Autodesk Inventor part; units mm, degrees
ref_plane "YZ Plane" through (0, 0, 0) normal (1, 0, 0) x (0, 1, 0)
ref_plane "XZ Plane" through (0, 0, 0) normal (0, 1, 0) x (-1, 0, 0)
ref_plane "XY Plane" through (0, 0, 0) normal (0, 0, 1) x (1, 0, 0)
sketch "Sketch1" plane through (0, 0, 0) normal (0, 1, 0) x (-1, 0, 0)
  line L0 (0, 0) -> (-20, 0)
  line L1 (-20, 0) -> (-20, -100)
  line L2 (-20, -100) -> (0, -100)
  line L3 (0, -100) -> (0, 0)
  dimension "d0" = 20
  dimension "d1" = 100
extrude "Extrusion1" add sketch "Sketch1" along normal blind 15
sketch "Sketch2" plane through (0, 15, 0) normal (0, 1, 0) x (1, 0, 0)
  line L0 (20, 0) -> (20, 100)
  line L1 (0, 100) -> (0, 0)
  line L2 (20, 0) -> (0, 0)
  line L3 (0, 0) -> (0, 19.5)
  line L4 (0, 19.5) -> (20, 19.5)
  line L5 (20, 19.5) -> (20, 0)
  dimension "d4" = 19.5
extrude "Extrusion2" add sketch "Sketch2" along normal blind 15
sketch "Sketch3" plane through (0, 15, 0) normal (0, 1, 0) x (1, 0, 0)
  line L0 (20, 19.5) -> (0, 19.5)
  line L1 (0, 19.5) -> (0, 22.5)
  line L2 (0, 100) -> (0, 0)
  line L3 (0, 22.5) -> (3.0005, 19.5)
  line L4 (3.0005, 19.5) -> (0, 19.5)
  line L5 (20, 19.5) -> (20, 22.5)
  line L6 (20, 0) -> (20, 100)
  line L7 (20, 22.5) -> (16.9995, 19.5)
  line L8 (16.9995, 19.5) -> (20, 19.5)
  dimension "d7" = 3
  dimension "d8" = 4.243
  dimension "d9" = 3
  dimension "d10" = 4.243
extrude "Extrusion3" add sketch "Sketch3" along normal blind 15
sketch "Sketch4" plane through (0, 0, 0) normal (0, 0, 1) x (1, 0, 0)
  point P0 (0, 0)
sketch "Sketch5" plane through (0, 0, 0) normal (0, 0, 1) x (1, 0, 0)
  line L0 (0, 0) -> (20, 0)
  line L1 (20, 30) -> (16.9995, 30)
  line L2 (0, 0) -> (20, 0)
  line L3 (20, 0) -> (20, 30)
  line L4 (20, 30) -> (0, 30)
  line L5 (0, 30) -> (0, 0)
extrude "Extrusion4" add sketch "Sketch5" along normal blind 80
sketch "Sketch6" plane through (0, 0, 80) normal (0, 0, 1) x (1, 0, 0)
  line L0 (19, 3) -> (1, 3)
  line L1 (1, 3) -> (1, 12)
  line L2 (1, 12) -> (19, 12)
  line L3 (19, 12) -> (19, 3)
  line L4 (0, 30) -> (0, 0)
  line L5 (0, 0) -> (20, 0)
  dimension "d15" = 18
  dimension "d16" = 9
  dimension "d17" = 1
  dimension "d18" = 3
extrude "Extrusion5" cut sketch "Sketch6" against normal blind 160
sketch "Sketch7" plane through (0, 0, 0) normal (0, -1, 0) x (1, 0, 0)
  circle A0 centre (10, -89.5) radius 2.25
  circle A1 centre (10, -74.5) radius 2.25
  line L0 (20, -100) -> (0, -100)
  line L1 (0, -100) -> (0, 80)
  point P0 (0, 0)
  point P1 (10, -100)
  dimension "d21" = 4.5
  dimension "d22" = 4.5
  dimension "d23" = 10.5
  dimension "d24" = 10.5
  dimension "d25" = 10
  dimension "d26" = 10
extrude "Extrusion6" cut sketch "Sketch7" against normal blind 160
sketch "Sketch8" plane through (0, 0, -80) normal (0, 0, 1) x (1, 0, 0)
  line L0 (19, 3) -> (1, 3)
  line L1 (1, 12) -> (19, 12)
  line L2 (19, 3) -> (1, 3)
  line L3 (1, 3) -> (1, 12)
  line L4 (1, 12) -> (19, 12)
  line L5 (19, 12) -> (19, 3)
  point P0 (0, 0)
extrude "Extrusion7" add sketch "Sketch8" along normal blind 170
sketch "Sketch9" plane through (0, 30, 0) normal (0, 1, 0) x (1, 0, 0)
  point P0 (0, 0)
sketch "Sketch10" plane through (0, 0, 90) normal (0, 0, 1) x (1, 0, 0)
  line L0 (19, 3) -> (1, 3)
  line L1 (1, 12) -> (19, 12)
  line L2 (1, 3) -> (19, 3)
  line L3 (19, 3) -> (19, 12)
  line L4 (19, 12) -> (1, 12)
  line L5 (1, 12) -> (1, 3)
  point P0 (0, 0)
extrude "Extrusion8" cut sketch "Sketch10" against normal blind 185
sketch "Sketch11" plane through (0, 15, 0) normal (0, 1, 0) x (1, 0, 0)
  line L0 (0, 100) -> (0, -80)
  line L1 (20, -80) -> (20, 100)
  line L2 (0, 100) -> (20, 100)
  line L3 (20, 100) -> (20, 97.7472)
  line L4 (20, 97.7472) -> (0, 97.7472)
  line L5 (0, 97.7472) -> (0, 100)
  point P0 (0, 0)
  point P1 (0, 97.7472)
extrude "Extrusion9" cut sketch "Sketch11" against normal blind 185
sketch "Sketch12" plane through (0, 30, 0) normal (0, 1, 0) x (1, 0, 0)
  circle A0 centre (10, -70.4515) radius 30
  point P0 (0, 0)
  dimension "d35" = 60
extrude "Extrusion10" add sketch "Sketch12" along normal mid plane 60
sketch "Sketch13" plane through (10, 60, 70.4515) normal (0, 1, 0) x (1, 0, 0)
  circle A0 centre (0, 0) radius 30
  point P0 (-10, 70.4515)
extrude "Extrusion11" cut sketch "Sketch13" against normal blind 30
sketch "Sketch14" plane through (0, 30, 0) normal (0, 1, 0) x (1, 0, 0)
  point P0 (0, 0)
sketch "Sketch15" plane through (0, 0, 0) normal (0, -1, 0) x (1, 0, 0)
  arc A0 (1, 41.8333) -> (19, 41.8333) centre (10, 70.4515) ccw
  circle A1 centre (4.9424, 40.8809) radius 2.5
  circle A2 centre (15.0576, 40.8809) radius 2.5
  point P0 (0, 0)
  dimension "d40" = 5
  dimension "d41" = 5
extrude "Extrusion12" cut sketch "Sketch15" against normal blind 13
sketch "Sketch16" plane through (0, 0, 0) normal (0, -1, 0) x (1, 0, 0)
  circle A0 centre (10, -89.5) radius 2.25
  circle A1 centre (10, -89.5) radius 3.5
  circle A2 centre (10, -74.5) radius 2.25
  circle A3 centre (10, -74.5) radius 3.5
  point P0 (0, 0)
  dimension "d44" = 7
  dimension "d45" = 7
extrude "Extrusion13" cut sketch "Sketch16" against normal blind 6
fillet "Fillet1" radius 2 8 edges at (20, 30, 9.8336) (20, 15, -60.1236) (0, 15, -60.1236) (0, 30, 9.8336) (0, 0, -27.79) (20, 0, -27.79) (10, 30, 100.4515) (10, 0, 100.4515)
sketch "Sketch17" plane through (0, 0, 0) normal (0, -1, 0) x (1, 0, 0)
  circle A0 centre (10, 22.1222) radius 2.4
  line L0 (2, -97.7472) -> (2, 43.6187)
  point P0 (0, 0)
  dimension "d49" = 4.8
  dimension "d50" = 8
extrude "Extrusion14" cut sketch "Sketch17" against normal blind 6
properties part number "shotHolder"
Geometry check sheet. Reference: the model listing, model coordinates, mm. A direction names the side the tool comes from. Round coordinates to 2 decimals unless told otherwise and drop trailing zeros. Order: outer loops, then holes, each group sorted by start corner. A loop starts at its lowest first (then second) coordinate and runs counter-clockwise, first axis right, second up. Notation, with made-up numbers: (-27.75, 87) - (-21.75, 87) arc R18 cw to (-21.75, 121) - close; hole circle Ø4 at (-5, -21). An arc over 180 degrees is marked (long way). Use a Markdown table: item, result. Add a question column.
1) Gauge pin test, flat ends, axial feed: P1, Ø5, axis at y = 3.5, z = -34.5, coming from the +X side; P2, Ø9, axis at x = 8, z = -49, coming from the +Y side; P3, Ø7, axis at x = 10, y = 21.5, coming from the -Z side. Record the tip position at first contact, or that the pin passes through.
2) Thickness scan on line 1 along Z through (x, y) = (10, 2); line 2 along Z through (x, y) = (10, 13); line 3 along Y through (x, z) = (16.5, -76). Record the ranges inside material, lowest first.
3) Section check A-A (x = 10). Count the separate pieces of the cut face and the enclosed holes in it, then the cut area to 3 significant figures.
4) Mould release check, pull along Z, two halves, no side actions. Record for faces 1 (the flat face through (20, 12, -13)), 2 (the flat face through (1, 8, -26)), 3 (the cylindrical face through (8.82, 15.18, 100.43)): released by +Z, released by -Z, zero draft, split by the parting line, or undercut.
5) Section check D-D (z = -13). Record the cut outline in (x, y), then the cut area to 3 significant figures.
6) Section check B-B (y = 9.5). Record the cut outline in (x, z), then the cut area to 3 significant figures.
7) Section check C-C (z = -89.5). Record the cut outline in (x, y), then the cut area to 3 significant figures.
8) Set-up check for faces 4 (the flat face through (10, 3, -26)), 5 (the cylindrical face through (9.241, 1.479, -92.917)), 6 (the flat face through (0, 12, -13)): record each of +Z, -Z, +X, -X, +Y, -Y from which the full face is reachable in a straight line by a thin tool's end or side.
Established:
| question | item | result |
|---|---|---|
| 1 | P1 | x = 20 |
| 1 | P2 | y = 15 |
| 1 | P3 | z = -19.5 |
| 2 | line 1 | -97.75 to -93, -86 to -78, -71 to 19.72, 24.52 to 100.45 |
| 2 | line 2 | -97.75 to -91.75, -87.25 to -76.75, -72.25 to 100.45 |
| 2 | line 3 | 0 to 3, 12 to 15 |
| 3 | separate pieces | 5 |
| 3 | enclosed holes | 0 |
| 3 | area | 3,470 mm2 |
| 4 | face 1 | zero draft |
| 4 | face 2 | undercut |
| 4 | face 3 | split by the parting line |
| 5 | outline | (0, 2) arc R2 ccw to (2, 0) - (18, 0) arc R2 ccw to (20, 2) - (20, 28) arc R2 ccw to (18, 30) - (2, 30) arc R2 ccw to (0, 28) - close; hole (1, 3) - (19, 3) - (19, 12) - (1, 12) - close |
| 5 | area | 435 mm2 |
| 6 | outline | (0, -97.75) - (20, -97.75) - (20, 42.17) arc R30 ccw (long way) to (0, 42.17) - close; hole (1, -95) - (19, -95) - (19, 41.83) arc R30 cw to (17.5, 41.4) arc R2.5 ccw to (12.58, 40.56) arc R30 cw to (7.42, 40.56) arc R2.5 ccw to (2.5, 41.4) arc R30 cw to (1, 41.83) - close |
| 6 | area | 3,140 mm2 |
| 7 | outline | (0, 2) arc R2 ccw to (2, 0) - (6.5, 0) - (6.5, 3) - (1, 3) - (1, 12) - (7.75, 12) - (7.75, 15) - (2, 15) arc R2 ccw to (0, 13) - close; (12.25, 12) - (19, 12) - (19, 3) - (13.5, 3) - (13.5, 0) - (18, 0) arc R2 ccw to (20, 2) - (20, 13) arc R2 ccw to (18, 15) - (12.25, 15) - close |
| 7 | area | 100 mm2 |
| 8 | face 4 | none |
| 8 | face 5 | -Y |
| 8 | face 6 | -Z, -X, +Y, -Y |
